Autodesk Inventor part; units mm, degrees
ref_plane "YZ Plane" through (0, 0, 0) normal (1, 0, 0) x (0, 1, 0)
ref_plane "XZ Plane" through (0, 0, 0) normal (0, 1, 0) x (-1, 0, 0)
ref_plane "XY Plane" through (0, 0, 0) normal (0, 0, 1) x (1, 0, 0)
sketch "Sketch1" plane through (0, 0, 0) normal (0, 0, 1) x (1, 0, 0)
  line L0 (0, 0) -> (-50.8, 0)
  line L1 (-50.8, 0) -> (-50.8, 57.15)
  line L2 (-50.8, 57.15) -> (0, 57.15)
  line L3 (0, 57.15) -> (0, 0)
  line L4 (-50.8, 0) -> (-50.8, 25.4)
  line L5 (0, 0) -> (0, 25.4)
  line L6 (-25.4, 57.15) -> (-38.1, 57.15)
  line L7 (-25.4, 57.15) -> (-12.7, 57.15)
  line L8 (-12.7, 57.15) -> (0, 28.575)
  line L9 (-38.1, 57.15) -> (-50.8, 25.4)
  dimension "d0" = 50.8
  dimension "d1" = 57.15
  dimension "d2" = 25.4
  dimension "d3" = 12.7
  dimension "d4" = 12.7
extrude "Extrusion1" add sketch "Sketch1" along normal blind 3.175 contours L0 L1 L9 L2 L8 L3
sketch "Sketch2" plane through (0, 0, 3.175) normal (0, 0, 1) x (1, 0, 0)
  line L0 (-12.7, 57.15) -> (-38.1, 57.15)
  line L1 (-50.8, 0) -> (0, 0)
  line L2 (-38.1, 57.15) -> (-38.1, 95.25)
  line L3 (-38.1, 95.25) -> (-12.7, 95.25)
  line L4 (-12.7, 95.25) -> (-12.7, 57.15)
  dimension "d7" = 38.1
extrude "Extrusion2" add sketch "Sketch2" against normal blind 3.175
sketch "Sketch3" plane through (0, 0, 0) normal (0, 0, -1) x (-1, 0, 0)
  circle A0 centre (25.4, 57.15) radius 3.3782
  circle A1 centre (25.4, 44.45) radius 3.3782
  circle A2 centre (25.4, 31.75) radius 3.3782
  circle A3 centre (12.7, 12.7) radius 3.302
  circle A4 centre (38.1, 12.7) radius 3.302
extrude "Extrusion3" cut sketch "Sketch3" against normal blind 3.175
sketch "Sketch4" plane through (0, 0, 3.175) normal (0, 0, 1) x (1, 0, 0)
  line L0 (-12.7, 95.25) -> (-38.1, 95.25)
  line L1 (-38.1, 95.25) -> (-34.29, 95.25)
  line L2 (-34.29, 95.25) -> (-34.29, 88.9)
  line L3 (-34.29, 88.9) -> (-34.29, 76.2)
  line L4 (-12.7, 95.25) -> (-16.51, 95.25)
  line L5 (-16.51, 95.25) -> (-16.51, 88.9)
  line L6 (-16.51, 88.9) -> (-16.51, 82.55)
  circle A0 centre (-34.29, 88.9) radius 3.3782
  circle A1 centre (-16.51, 88.9) radius 3.3782
  circle A2 centre (-34.29, 76.2) radius 3.3782
  line L7 (-16.51, 88.9) -> (-16.51, 76.2)
  circle A3 centre (-16.51, 76.2) radius 3.3782
  dimension "d12" = 3.81
  dimension "d13" = 6.35
  dimension "d14" = 12.7
  dimension "d15" = 3.81
  dimension "d16" = 6.7564
  dimension "d17" = 6.7564
  dimension "d18" = 6.7564
  dimension "d19" = 6.7564
extrude "Extrusion4" cut sketch "Sketch4" against normal blind 25.4
sketch "Sketch5" plane through (-12.7, 57.15, 3.175) normal (1, 0, 0) x (0, 0, -1)
  line L0 (0, 0) -> (0, 38.1)
  line L1 (3.175, 0) -> (0, 0)
  line L2 (3.175, 38.1) -> (3.175, 0)
  line L3 (0, 38.1) -> (3.175, 38.1)
  point P0 (3.175, -57.15)
extrude "Extrusion5" add sketch "Sketch5" along normal blind 3.175
sketch "Sketch6" plane through (-38.1, 57.15, 3.175) normal (-1, 0, 0) x (0, 0, 1)
  line L0 (0, 38.1) -> (0, 0)
  line L1 (0, 38.1) -> (-3.175, 38.1)
  line L2 (-3.175, 0) -> (-3.175, 38.1)
  line L3 (-3.175, 0) -> (0, 0)
  point P0 (-3.175, -57.15)
extrude "Extrusion6" add sketch "Sketch6" along normal blind 3.175
properties part number "that thing mount" material "Aluminum 6061"
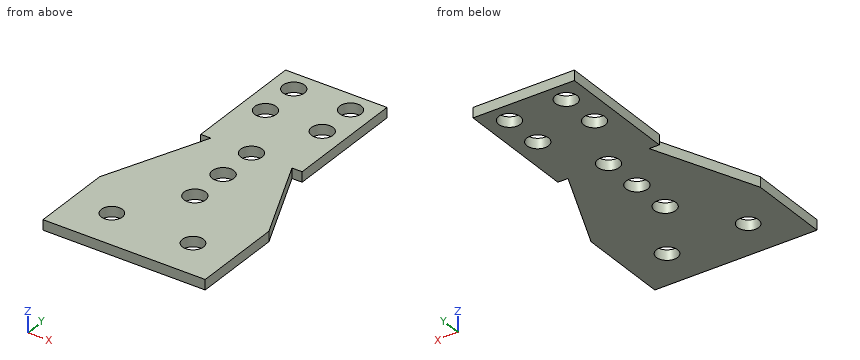
Can you work these out from the model? Positions are in its coordinate system, mm. Coordinates: 2 decimals unless noted, no trailing zeros. Write each loop counter-clockwise with the first axis right and the second up, starting at its lowest first coordinate (ties: lowest second). Pieces come first, ordered by that corner, then holes. Notation, with made-up numbers: (5, 86.25) - (48, 86.25) arc R32 ccw to (48, 112.25) - close; hole circle Ø7 at (84.5, 68.5). An arc over 180 degrees is marked (long way). Return JSON: item names as keys, results as strings.
Q1. If we section it at A-A (x = -25.4): Please give me the cut outline in (y, z) (3 decimals), then the cut area to 3 significant figures.
Computed values:
{"outline": "(0, 0) - (28.372, 0) - (28.372, 3.175) - (0, 3.175) - close; (35.128, 0) - (41.072, 0) - (41.072, 3.175) - (35.128, 3.175) - close; (47.828, 0) - (53.772, 0) - (53.772, 3.175) - (47.828, 3.175) - close; (60.528, 0) - (95.25, 0) - (95.25, 3.175) - (60.528, 3.175) - close", "area": "238 mm2"}
Q2. I'm going to push flat-ended pins straight in: pin 1 Ø1 at (y, z) = (78, 2.5) entering from -X (3 decimals); pin 2 Ø6 at (x, y) = (-34.29, 88.9) entering from +Z. Where does each tip first touch, or does it pass through?
Computed values:
{"pin 1": "stops at x = -41.275", "pin 2": "passes through"}
Q3. If we section it at C-C (z = 1.35): Count the separate pieces of the cut face and the enclosed holes in it, then the cut area to 3 significant figures.
Computed values:
{"separate pieces": "1", "enclosed holes": "9", "area": "3,410 mm2"}
Q4. Please list where these lines run through material, in increasing order: L1, parallel to Y at x = -25.4, z = 1.6; L2, parallel to X at y = 88.9, z = 1.9 (3 decimals); L3, parallel to X at y = 13, z = 2.9. Write a range as from..to.
Computed values:
{"L1": "y = 0..28.37, 35.13..41.07, 47.83..53.77, 60.53..95.25", "L2": "x = -41.275..-37.668, -30.912..-19.888, -13.132..-9.525", "L3": "x = -50.8..-41.39, -34.81..-15.99, -9.41..0"}
Q5. If we section it at B-B (y = 10.5): Please give me the cut outline in (x, z) (3 decimals), then the cut area to 3 significant figures.
Computed values:
{"outline": "(-50.8, 0) - (-40.562, 0) - (-40.562, 3.175) - (-50.8, 3.175) - close; (-35.638, 0) - (-15.162, 0) - (-15.162, 3.175) - (-35.638, 3.175) - close; (-10.238, 0) - (0, 0) - (0, 3.175) - (-10.238, 3.175) - close", "area": "130 mm2"}
Q6. If we section it at D-D (x = -40): Please give me the cut outline in (y, z) (3 decimals).
Computed values:
{"outline": "(0, 0) - (9.999, 0) - (9.999, 3.175) - (0, 3.175) - close; (15.401, 0) - (52.4, 0) - (52.4, 3.175) - (15.401, 3.175) - close; (57.15, 0) - (95.25, 0) - (95.25, 3.175) - (57.15, 3.175) - close"}
